Design review of the part shown in the three views and the two pictorial views. Dimensions are in mm from the part's minimum x, y and z. Give positions to 0.01 mm unless a question says otherwise; leave off trailing zeros. Order: outer loops, then holes, each group sorted by start corner. A loop starts at its lowest first (then second) coordinate and runs counter-clockwise, first axis right, second up.
Item 1: For P1, Ø6.5, axis at x = 6.5, y = 69, coming from the +Z side, flat-tipped, find the tip position at first contact; note if it passes through.
Item 2: Consider section B-B (y = 69). Give the boundary of the cut face in (x, z), plus the area to 3 significant figures.
Item 3: Consider section C-C (z = 4.5). Give the boundary of the cut face in (x, y).
Item 4: For probe 1 along Y at (x, z) = (6.5, 8); probe 2 along X at (y, z) = (71.5, 5.5); probe 3 along Y at (x, z) = (4, 4.5), list the stretches that pass through material, from the lowest coordinate up.
Item 5: Consider section A-A (x = 47.5). Give the boundary of the cut face in (y, z).
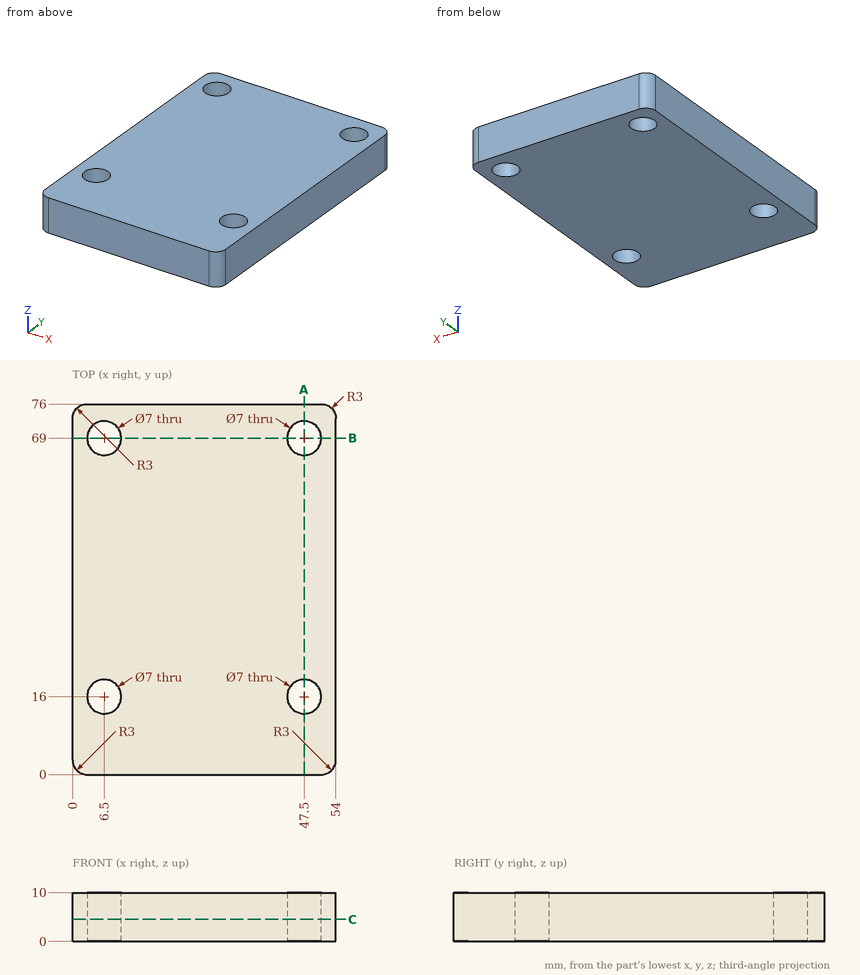
Resolved:
1. P1: passes through
2. outline: (0, 0) - (3, 0) - (3, 10) - (0, 10) - close; (10, 0) - (44, 0) - (44, 10) - (10, 10) - close; (51, 0) - (54, 0) - (54, 10) - (51, 10) - close
2. area: 400 mm2
3. outline: (0, 3) arc R3 ccw to (3, 0) - (51, 0) arc R3 ccw to (54, 3) - (54, 73) arc R3 ccw to (51, 76) - (3, 76) arc R3 ccw to (0, 73) - close; hole circle Ø7 at (6.5, 16); hole circle Ø7 at (6.5, 69); hole circle Ø7 at (47.5, 16); hole circle Ø7 at (47.5, 69)
4. probe 1: y = 0 to 12.5, 19.5 to 65.5, 72.5 to 76
4. probe 2: x = 0 to 4.05, 8.95 to 45.05, 49.95 to 54
4. probe 3: y = 0 to 13.55, 18.45 to 66.55, 71.45 to 76
5. outline: (0, 0) - (12.5, 0) - (12.5, 10) - (0, 10) - close; (19.5, 0) - (65.5, 0) - (65.5, 10) - (19.5, 10) - close; (72.5, 0) - (76, 0) - (76, 10) - (72.5, 10) - close
